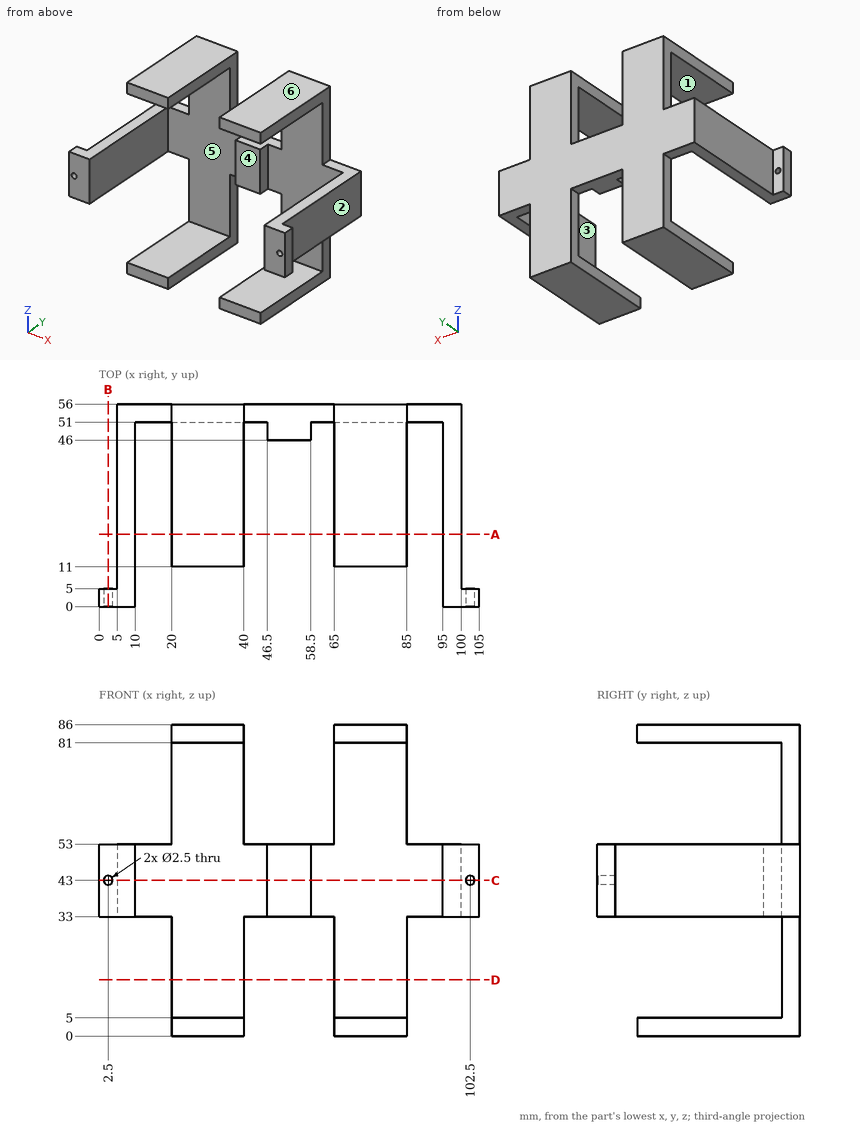
The drawing under review shows one solid part. Ordinate dimensions are in mm from its lowest x, y, z. A direction names the side the tool comes from. Coordinates: 2 decimals unless noted, no trailing zeros. Write each loop counter-clockwise with the first axis right and the second up, starting at its lowest first coordinate (ties: lowest second). Pieces come first, ordered by that corner, then holes. Notation, with made-up numbers: (83.25, 70) - (130.25, 70) arc R15 ccw to (130.25, 83) - close; hole circle Ø9 at (-35.75, 39.5). An arc over 180 degrees is marked (long way). Put each result on its own line as item: value.
1. Add section D-D, the plane z = 15.5. Give the boundary of the cut face in (x, y), then the cut area to 3 significant figures.
Values found:
outline: (20, 51) - (40, 51) - (40, 56) - (20, 56) - close; (65, 51) - (85, 51) - (85, 56) - (65, 56) - close
area: 200 mm²
2. Wall thickness on probe 1 along Z at (x, y) = (73.5, 41); probe 2 along X at (y, z) = (5.5, 38); probe 3 along Y at (x, z) = (47.5, 42.5): over which ranges is each line inside the solid? List them lowest first.
Values found:
probe 1: 0 to 5, 81 to 86
probe 2: 5 to 10, 95 to 100
probe 3: 46 to 56
3. For pin 1 (11 mm diameter, centred on x = 72, z = 46, fed in from -Y); pin 2 (6 mm diameter, centred on x = 9, y = 16.5, fed in from -Z); pin 3 (4 mm diameter, centred on y = 48.5, z = 42.5, fed in from +X); pin 4 (10 mm diameter, centred on x = 25.5, y = 39.5, fed in from -Z), all flat-tipped, find the tip position at first contact; note any pin that passes through.
Values found:
pin 1: y = 51
pin 2: z = 33
pin 3: x = 100
pin 4: z = 0
4. Add section A-A, the plane y = 20. Give the boundary of the cut face in (x, z).
Values found:
outline: (5, 33) - (10, 33) - (10, 53) - (5, 53) - close; (20, 0) - (40, 0) - (40, 5) - (20, 5) - close; (20, 81) - (40, 81) - (40, 86) - (20, 86) - close; (65, 0) - (85, 0) - (85, 5) - (65, 5) - close; (65, 81) - (85, 81) - (85, 86) - (65, 86) - close; (95, 33) - (100, 33) - (100, 53) - (95, 53) - close
5. Add section C-C, the plane z = 43. Give the boundary of the cut face in (x, y).
Values found:
outline: (0, 0) - (1.25, 0) - (1.25, 5) - (0, 5) - close; (3.75, 0) - (10, 0) - (10, 51) - (46.5, 51) - (46.5, 46) - (58.5, 46) - (58.5, 51) - (95, 51) - (95, 0) - (101.25, 0) - (101.25, 5) - (100, 5) - (100, 56) - (5, 56) - (5, 5) - (3.75, 5) - close; (103.75, 0) - (105, 0) - (105, 5) - (103.75, 5) - close
6. Add section B-B, the plane x = 2.5. Give the boundary of the cut face in (y, z).
Values found:
outline: (0, 33) - (5, 33) - (5, 41.75) - (0, 41.75) - close; (0, 44.25) - (5, 44.25) - (5, 53) - (0, 53) - close
7. Mouldability with a two-part tool opening along Z and no side actions: class the marked faces 4, 5 and 6 as released by +Z, released by -Z, zero draft, split by the parting line, or undercut.
Values found:
face 4: zero draft
face 5: undercut
face 6: released by +Z
8. Machinability: for the marked faces 1, 2 and 3, which of the approach directions +Z, -Z, +X, -X, +Y, -Y give a long, thin tool a straight path to every point of the face, cutting with its end or side? Answer none if there is none.
Values found:
face 1: +X, -X, -Y
face 2: +Z, -Z, +X, +Y
face 3: +Z, -Z, -Y
